```python
from build123d import *

# Parameters (mm, degrees)
PAD_DEPTH       = 23.5
SKETCH014_W     = 8
SKETCH014_H     = 0.8
POCKET001_DEPTH = 0.7
SKETCH015_W     = 5.25
SKETCH015_H     = 1
POCKET002_DEPTH = 0.5
SKETCH020_R     = 3.4
POCKET005_DEPTH = 1.5
POCKET006_DEPTH = 1.5
SKETCH025_R     = 3.1
POCKET008_DEPTH = 16.5
PAD015_DEPTH    = 15.75


with BuildPart() as part:
    # Sketch → Pad (new body)
    with BuildSketch(Plane.XY.offset(6)):
        with BuildLine():
            Line((-29.25, 12.75), (29.25, 12.75))
            ThreePointArc((33, 9), (31.9016504294, 11.6516504294), (29.25, 12.75))
            Line((33, 9), (33, -9))
            ThreePointArc((29.25, -12.75), (31.9016504295, -11.6516504294), (33, -9))
            Line((29.25, -12.75), (-29.25, -12.75))
            ThreePointArc((-33, -9), (-31.9016504294, -11.6516504295), (-29.25, -12.75))
            Line((-33, -9), (-33, 9))
            ThreePointArc((-29.25, 12.75), (-31.9016504294, 11.6516504294), (-33, 9))
        make_face()
        with BuildLine():
            Line((-29.25, 11.25), (29.25, 11.25))
            ThreePointArc((31.5, 9), (30.8409902577, 10.5909902577), (29.25, 11.25))
            Line((31.5, 9), (31.5, -9))
            ThreePointArc((29.25, -11.25), (30.8409902577, -10.5909902577), (31.5, -9))
            Line((29.25, -11.25), (-29.25, -11.25))
            ThreePointArc((-31.5, -9), (-30.8409902577, -10.5909902577), (-29.25, -11.25))
            Line((-31.5, -9), (-31.5, 9))
            ThreePointArc((-29.25, 11.25), (-30.8409902577, 10.5909902577), (-31.5, 9))
        make_face(mode=Mode.SUBTRACT)
    extrude(amount=-PAD_DEPTH)

    # Sketch014 → Pocket001 (cut)
    with BuildSketch(Plane(origin=(0, -11.25, 6), x_dir=(-1, 0, 0), z_dir=(0, 1, 0))):
        with Locations((0, -21.9)):
            Rectangle(SKETCH014_W, SKETCH014_H)
    extrude(amount=-POCKET001_DEPTH, mode=Mode.SUBTRACT)

    # Sketch015 → Pocket002 (cut)
    with BuildSketch(Plane(origin=(0, 11.25, 6), x_dir=(1, 0, 0), z_dir=(0, -1, 0))):
        with Locations((-10.475, -22.55)):
            Rectangle(SKETCH015_W, SKETCH015_H)
        with Locations((10.475, -22.55)):
            Rectangle(SKETCH015_W, SKETCH015_H)
    extrude(amount=-POCKET002_DEPTH, mode=Mode.SUBTRACT)

    # Sketch020 → Pocket005 (cut)
    with BuildSketch(Plane(origin=(33, 0, 6), x_dir=(0, 1, 0), z_dir=(1, 0, 0))):
        with Locations((0, -14)):
            Circle(SKETCH020_R)
    extrude(amount=-POCKET005_DEPTH, mode=Mode.SUBTRACT)

    # Sketch022 → Pocket006 (cut)
    with BuildSketch(Plane(origin=(0, -12.75, 6), x_dir=(1, 0, 0), z_dir=(0, -1, 0))):
        with BuildLine():
            ThreePointArc((12.4, -2.8), (15, -5.4), (17.6, -2.8))
            Line((17.6, -2.8), (18.6, -2.8))
            Line((18.6, -2.8), (18.6, 0.1))
            Line((11.4, 0.1), (18.6, 0.1))
            Line((11.4, -2.8), (11.4, 0.1))
            Line((12.4, -2.8), (11.4, -2.8))
        make_face()
    extrude(amount=-POCKET006_DEPTH, mode=Mode.SUBTRACT)

    # Sketch025 → Pocket008 (cut)
    with BuildSketch(Plane(origin=(0, 0, -17.5), x_dir=(1, 0, 0), z_dir=(0, 0, -1))):
        with Locations((-20, -9)):
            Circle(SKETCH025_R)
    extrude(amount=-POCKET008_DEPTH, mode=Mode.SUBTRACT)

    # Sketch026 → Pad015 (new body)
    with BuildSketch(Plane(origin=(0, 0, -1), x_dir=(1, 0, 0), z_dir=(0, 0, -1))):
        with BuildLine():
            Line((-15, -6.5), (-18.252859479, -6.5))
            ThreePointArc((-16.95, -9), (-17.2952561499, -7.5904395346), (-18.252859479, -6.5))
            ThreePointArc((-18.252859479, -11.5), (-17.2952561499, -10.4095604654), (-16.95, -9))
            Line((-18.252859479, -11.5), (-15, -11.5))
            Line((-15, -6.5), (-15, -11.5))
        make_face()
        with BuildLine():
            Line((-25, -11.5), (-21.747140521, -11.5))
            ThreePointArc((-23.05, -9), (-22.7047438501, -10.4095604654), (-21.747140521, -11.5))
            ThreePointArc((-21.747140521, -6.5), (-22.7047438501, -7.5904395346), (-23.05, -9))
            Line((-21.747140521, -6.5), (-25, -6.5))
            Line((-25, -6.5), (-25, -11.5))
        make_face()
    extrude(amount=PAD015_DEPTH)


solid = part.part
```
Check sheet for the modelled part. Datum: model origin and axes. Units: mm. A direction names the side the tool comes from. Round coordinates to 2 decimals unless told otherwise and drop trailing zeros. Loops run counter-clockwise (first coordinate to the right, second up) from the corner with the lowest first, then second, coordinate; pieces in that order, holes last. Notation, with made-up numbers: (-7.5, -24.5) - (22.5, -24.5) arc R26 cw to (22.5, -6.5) - close; hole circle Ø5 at (37.5, 10.5). An arc over 180 degrees is marked (long way). Answer as a JSON object with one key per item and string values. Group by question number.
Q1. Sectioned sample at A-A, the plane x = -2. Enter the section's corners in (y, z), plus the area to 3 significant figures.
Q2. Sectioned sample at C-C, the plane z = -2.5. Enter the section's corners in (x, y), plus the area to 3 significant figures.
Q3. Gauge pin test, flat ends, axial feed: P1, Ø2.5, axis at x = -22.5, y = 8.5, coming from the +Z side; P2, Ø1, axis at x = -23, y = 8, coming from the -Z side; P3, Ø0.8, axis at y = -12, z = 5, coming from the -X side. Record the tip position at first contact, or that the pin passes through.
Q4. Mould release check, pull along Z, two halves, no side actions. Record for faces 1 (the face through (-16, 9, -16.75)), 2 (the face through (-16, 9, -1)), 3 (the face through (32.26, -0.74, -11.32)), 4 (the face through (-31.872, 11.681, -5.586)): released by +Z, released by -Z, zero draft, split by the parting line, or undercut.
Q5. Set-up check for faces 5 (the face through (0, -11.25, -6)), 6 (the face through (0.2, 11.4, -17.5)), 7 (the face through (18.6, -12, 5)): record each of +Z, -Z, +X, -X, +Y, -Y from which the full face is reachable in a straight line by a thin tool's end or side.
Q6. Sectioned sample at D-D, the plane y = -6.75. Enter the section's corners in (x, z).
Q7. Sectioned sample at B-B, the plane y = 0. Enter the section's corners in (x, z), plus the area to 3 significant figures.
Q8. Scan lines: line 1 along X through (y, z) = (9.25, -3.25); line 2 along Z through (x, y) = (32.2, 0); line 3 along X through (y, z) = (-3.75, -12). Record each from-to range of solid material in increasing order. Write a range as [from, to].
Solution:
{
 "1": {"outline": "(-12.75, -17.5) - (-11.25, -17.5) - (-11.25, -16.3) - (-11.95, -16.3) - (-11.95, -15.5) - (-11.25, -15.5) - (-11.25, 6) - (-12.75, 6) - close; (11.25, -17.5) - (12.75, -17.5) - (12.75, 6) - (11.25, 6) - close", "area": "69.9 mm²"},
 "2": {"outline": "(-33, -9) arc R3.75 ccw to (-29.25, -12.75) - (29.25, -12.75) arc R3.75 ccw to (33, -9) - (33, 9) arc R3.75 ccw to (29.25, 12.75) - (-29.25, 12.75) arc R3.75 ccw to (-33, 9) - close; hole (-31.5, -9) arc R2.25 ccw to (-29.25, -11.25) - (29.25, -11.25) arc R2.25 ccw to (31.5, -9) - (31.5, 9) arc R2.25 ccw to (29.25, 11.25) - (-15, 11.25) - (-15, 6.5) - (-18.25, 6.5) arc R3.05 ccw to (-18.25, 11.5) - (-18.17, 11.5) arc R3.1 ccw to (-21.83, 11.5) - (-21.75, 11.5) arc R3.05 ccw to (-21.75, 6.5) - (-25, 6.5) - (-25, 11.25) - (-29.25, 11.25) arc R2.25 ccw to (-31.5, 9) - close", "area": "277 mm²"},
 "3": {"P1": "stops at z = -1", "P2": "stops at z = -16.75", "P3": "stops at x = -31.95"},
 "4": {"face 1": "released by -Z", "face 2": "released by +Z", "face 3": "undercut", "face 4": "zero draft"},
 "5": {"face 5": "+Z, -Z", "face 6": "-Z, +X, -X, +Y, -Y", "face 7": "+Z, -Y"},
 "6": {"outline": "(-33, -17.5) - (-31.5, -17.5) - (-31.5, 6) - (-33, 6) - close; (31.5, -17.5) - (33, -17.5) - (33, 6) - (31.5, 6) - close"},
 "7": {"outline": "(-33, -17.5) - (-31.5, -17.5) - (-31.5, 6) - (-33, 6) - close; (31.5, -17.5) - (33, -17.5) - (33, -11.4) - (31.5, -11.4) - close; (31.5, -4.6) - (33, -4.6) - (33, 6) - (31.5, 6) - close", "area": "60.3 mm²"},
 "8": {"line 1": "x = [-32.99, -31.49], [-25, -23.04], [-16.96, -15], [31.49, 32.99]", "line 2": "z = [-17.5, -11.4], [-4.6, 6]", "line 3": "x = [-33, -31.5], [31.5, 33]"}
}
